Geometry: final body of the model. Coordinates: model frame, mm. Face numbers are marked on the shaded views. A direction names the side the tool comes from. Give positions to 0.01 mm unless a question says otherwise; leave off trailing zeros. Write each loop counter-clockwise with the first axis right and the second up, starting at its lowest first coordinate (ties: lowest second). Pieces come first, ordered by that corner, then holes.
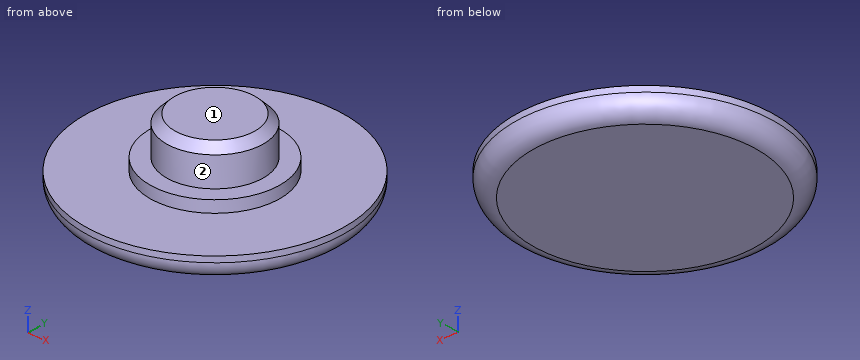
```python
from build123d import *

# Parameters (mm, degrees)
F0_R     = 11
F1_DEPTH = 2
F2_R     = 5.5
F3_DEPTH = 1
F4_R     = 4.1
F5_DEPTH = 3.2
F6_R     = 1.5
F7_SIZE  = 0.7


with BuildPart() as f1:
    # F0 (on Top) → F1 (new body)
    with BuildSketch(Plane.XY):
        Circle(F0_R)
    extrude(amount=F1_DEPTH)

    # F2 (on face) → F3 (join)
    with BuildSketch(Plane.XY.offset(2)):
        Circle(F2_R)
    extrude(amount=F3_DEPTH)

    # F4 (on face) → F5 (join)
    with BuildSketch(Plane.XY.offset(3)):
        Circle(F4_R)
    extrude(amount=F5_DEPTH)

    # F6
    f6_edges = [f1.edges().sort_by_distance(p)[0] for p in [
        (-11, 0, 0),
    ]]
    fillet(f6_edges, radius=F6_R)

    # F7
    f7_edges = [f1.edges().sort_by_distance(p)[0] for p in [
        (-4.1, 0, 6.2),
    ]]
    chamfer(f7_edges, length=F7_SIZE)


solid = f1.part
```
Item 1: Pin query (flat end, axial travel): pin 1 Ø1.5 at (x, y) = (0.5, 6) entering from +Z; pin 2 Ø1 at (x, z) = (-0.5, 4) entering from +Y. Return the tip coordinate at first contact, or that it passes through.
Found:
pin 1: stops at z = 3
pin 2: stops at y = 4.1
Item 2: Section D-D, the plane z = 1. Return the cut outline in (x, y).
Found:
outline: circle Ø21.83 at (0, 0)
Item 3: Section C-C, the plane z = 2.5. Return the cut outline in (x, y).
Found:
outline: circle Ø11 at (0, 0)
Item 4: Line query: L1, parallel to Z at x = -8.5, y = -3.75; L2, parallel to Z at x = -1.5, y = 5; L3, parallel to Y at x = 0.25, z = 5.25. Output: solid intervals per line, ascending.
Found:
L1: z = 0 to 2
L2: z = 0 to 3
L3: y = -4.09 to 4.09
Item 5: Section A-A, the plane y = 0. Return the cut outline in (x, z).
Found:
outline: (-11, 1.5) arc R1.5 ccw to (-9.5, 0) - (9.5, 0) arc R1.5 ccw to (11, 1.5) - (11, 2) - (5.5, 2) - (5.5, 3) - (4.1, 3) - (4.1, 5.5) - (3.4, 6.2) - (-3.4, 6.2) - (-4.1, 5.5) - (-4.1, 3) - (-5.5, 3) - (-5.5, 2) - (-11, 2) - close
Item 6: Reachability of the marked faces 1 and 2 from +Z, -Z, +X, -X, +Y, -Y: full face, straight path, thin tool, end or side. Return the list, or none.
Found:
face 1: +Z, +X, -X, +Y, -Y
face 2: +Z
